Read the model definition and answer for the solid it produces. Units are mm, in the model's axes. Face numbers are marked on the shaded views. A direction names the side the tool comes from. Coordinates: 2 decimals unless noted, no trailing zeros. Write each loop counter-clockwise with the first axis right and the second up, starting at its lowest first coordinate (ties: lowest second). Pieces come first, ordered by that corner, then holes.
from build123d import *

# Parameters (mm, degrees)
SKETCH_1_R             = 30
SKETCH_1_R_2           = 2.75
SKETCH_1_R_3           = 2.51
EXTRUDE_1_DEPTH        = 5
EXTRUDE_2_DEPTH        = 20
HOLE_WIZARD_M3_1_D     = 2.5
HOLE_WIZARD_M3_1_DEPTH = 5.6
CUT_EXTRUDE_1_REACH    = 57.616
SKETCH_5_R             = 1.6


with BuildPart() as part:
    # 草图1 → 凸台-拉伸1 (new body)
    with BuildSketch(Plane(origin=(0, 0, 0), x_dir=(1, 0, 0), z_dir=(0, 1, 0))):
        with Locations(Location((0, 0, 0), (0, 0, 270))):
            Circle(SKETCH_1_R)
        with Locations(Location((0, 22.5, 0), (0, 0, 270))):
            Circle(SKETCH_1_R_2, mode=Mode.SUBTRACT)
        with Locations(Location((19.485571585, 11.25, 0), (0, 0, 270))):
            Circle(SKETCH_1_R_2, mode=Mode.SUBTRACT)
        with Locations(Location((19.485571585, -11.25, 0), (0, 0, 270))):
            Circle(SKETCH_1_R_2, mode=Mode.SUBTRACT)
        with Locations(Location((0, -22.5, 0), (0, 0, 270))):
            Circle(SKETCH_1_R_2, mode=Mode.SUBTRACT)
        with Locations(Location((-19.485571585, -11.25, 0), (0, 0, 270))):
            Circle(SKETCH_1_R_2, mode=Mode.SUBTRACT)
        with Locations(Location((-19.485571585, 11.25, 0), (0, 0, 270))):
            Circle(SKETCH_1_R_2, mode=Mode.SUBTRACT)
        with Locations(Location((0, 0, 0), (0, 0, 270))):
            Circle(SKETCH_1_R_3, mode=Mode.SUBTRACT)
    extrude(amount=EXTRUDE_1_DEPTH)

    # 草图2 → 凸台-拉伸2 (add)
    with BuildSketch(Plane(origin=(0, 5, 0), x_dir=(1, 0, 0), z_dir=(0, 1, 0))):
        with BuildLine():
            Line((-7.2, 9.6), (7.2, 9.6))
            ThreePointArc((7.2, 9.6), (0, -12), (-7.2, 9.6))
        make_face()
        with BuildLine():
            Line((3, 4), (-3, 4))
            ThreePointArc((-3, 4), (0, -5), (3, 4))
        make_face(mode=Mode.SUBTRACT)
    extrude(amount=EXTRUDE_2_DEPTH)

    # M3 螺纹孔1
    with Locations(Plane(origin=(0, 0, -9.6), x_dir=(-1, 0, 0), z_dir=(0, 0, -1))):
        with Locations((0, 21)):
            Hole(HOLE_WIZARD_M3_1_D / 2, depth=HOLE_WIZARD_M3_1_DEPTH)

    # 草图5 → 切除-拉伸1 (cut, up to next)
    with BuildSketch(Plane(origin=(0, 0, -9.6), x_dir=(-1, 0, 0), z_dir=(0, 0, -1)), mode=Mode.PRIVATE) as cut_extrude_1_sk1:
        with Locations((0, 15)):
            Circle(SKETCH_5_R)
    cut_extrude_1_tool1 = extrude(cut_extrude_1_sk1.sketch, amount=-CUT_EXTRUDE_1_REACH, mode=Mode.PRIVATE) & part.part
    add(cut_extrude_1_tool1.solids().sort_by_distance((0, 15, -9.6))[0], mode=Mode.SUBTRACT)


solid = part.part
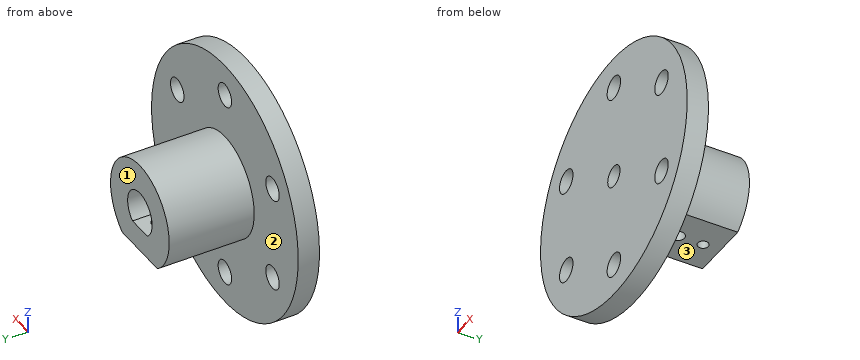
Item 1: The part is cut by section C-C (y = 4). Give the vertices of the cut face in (x, z), and give its area (3 significant figures).
Item 2: Given pin 1 (1.5 mm diameter, centred on x = -7.5, y = 21.5, fed in from +Z); pin 2 (3 mm diameter, centred on x = -0.5, y = 18.5, fed in from +Z); pin 3 (9 mm diameter, centred on x = 0, z = 22.5, fed in from -Y); pin 4 (7 mm diameter, centred on x = 19.49, z = -11.25, fed in from +Y), each flat-ended and moving along its own axis, determine where each tip first touches the part or whether it passes through.
Item 3: The part is cut by section B-B (x = 0). State how many separate pieces and enclosed holes the cut face has, and give its area (3 significant figures).
Item 4: The part is cut by section A-A (z = 0). Give the vertices of the cut face in (x, y).
Item 5: Find the intervals of material crossed by probe 1 along X at (y, z) = (2.85, 0); probe 2 along Z at (x, y) = (0, 10.5); probe 3 along Y at (x, z) = (-20.5, 2.5), in increasing order.
Item 6: For the marked faces 1, 2 and 3, determine the directions among +Z, -Z, +X, -X, +Y, -Y from which every point of the face is accessible in a straight line to the end or side of a thin tool.
Item 7: The part is cut by section D-D (z = 11.25). Give the vertices of the cut face in (x, y).
Answer:
1. outline: circle Ø60 at (0, 0); hole circle Ø5.5 at (-19.49, -11.25); hole circle Ø5.5 at (-19.49, 11.25); hole circle Ø5.5 at (0, -22.5); hole circle Ø5.5 at (0, 22.5); hole circle Ø5.02 at (0, 0); hole circle Ø5.5 at (19.49, -11.25); hole circle Ø5.5 at (19.49, 11.25)
1. area: 2,670 mm2
2. pin 1: stops at z = 9.92
2. pin 2: stops at z = 12
2. pin 3: stops at y = 0
2. pin 4: stops at y = 5
3. separate pieces: 6
3. enclosed holes: 0
3. area: 440 mm2
4. outline: (-30, 0) - (-2.51, 0) - (-2.51, 5) - (-5, 5) - (-5, 25) - (-12, 25) - (-12, 5) - (-30, 5) - close; (2.51, 0) - (30, 0) - (30, 5) - (12, 5) - (12, 25) - (5, 25) - (5, 5) - (2.51, 5) - close
5. probe 1: x = -30 to -2.51, 2.51 to 30
5. probe 2: z = -9.6 to -4, 5 to 12
5. probe 3: y = 0 to 5
6. face 1: +Z, -Z, +X, -X, +Y
6. face 2: +Y
6. face 3: -Z, +X, -X, +Y
7. outline: (-27.81, 0) - (-22.24, 0) - (-22.24, 5) - (-27.81, 5) - close; (-16.74, 0) - (16.74, 0) - (16.74, 5) - (4.18, 5) - (4.18, 25) - (-4.18, 25) - (-4.18, 5) - (-16.74, 5) - close; (22.24, 0) - (27.81, 0) - (27.81, 5) - (22.24, 5) - close
